Design review of the part shown in the three views and the two pictorial views. Dimensions are in mm from the part's minimum x, y and z. A direction names the side the tool comes from. Give positions to 0.01 mm unless a question says otherwise; leave off trailing zeros. Write each loop counter-clockwise with the first axis right and the second up, starting at its lowest first coordinate (ties: lowest second). Pieces come first, ordered by that corner, then holes. Notation, with made-up numbers: (27.5, 32) -> (59.5, 32) arc R27 ccw to (59.5, 64) -> close; hole circle Ø3 at (13, 13.25). An arc over 180 degrees is marked (long way). Use CSV: the item, a comma, the result in double quotes.
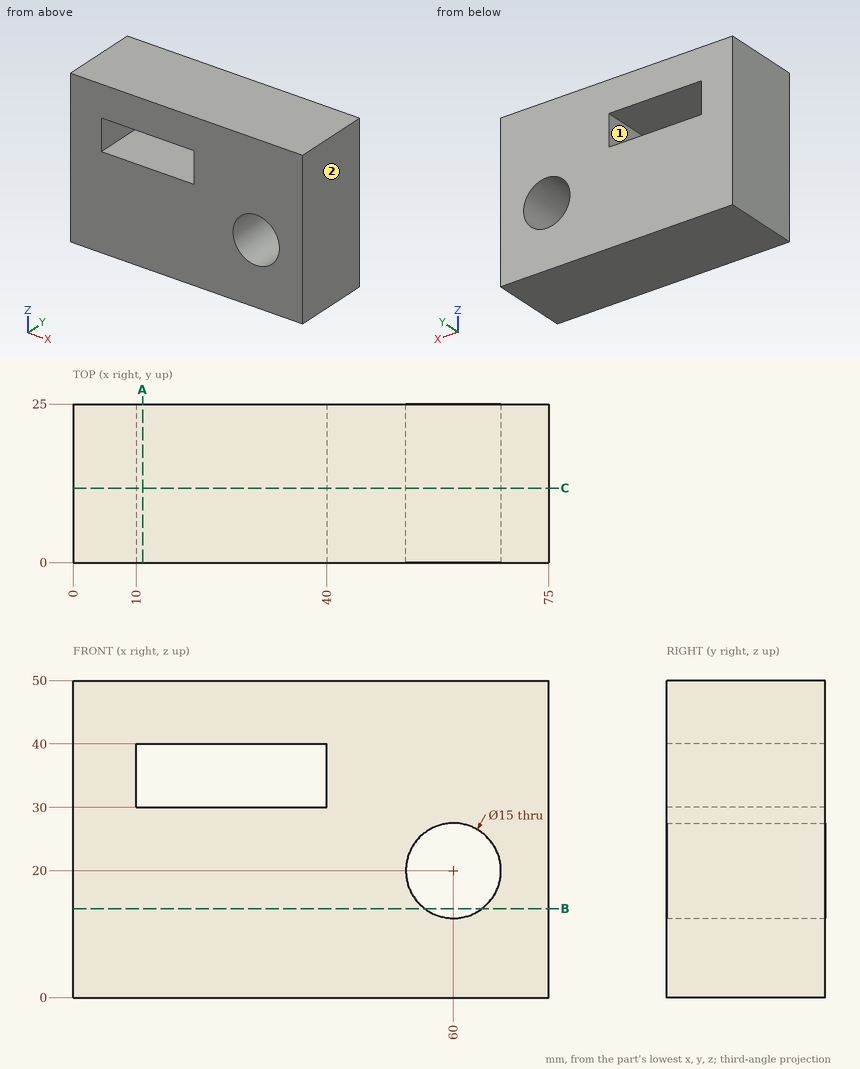
Q1. Insertion check: pin 1 (4 mm diameter, centred on x = 19.5, z = 7.5, fed in from -Y). The pin has a flat end and moves straight along its axis. Give the tip position at first contact, or say it passes through.
Derived:
pin 1,"stops at y = 0"
Q2. Consider section C-C (y = 11.75). Write out the cut boundary in (x, z).
Derived:
outline,"(0, 0) -> (75, 0) -> (75, 50) -> (0, 50) -> close; hole (10, 30) -> (40, 30) -> (40, 40) -> (10, 40) -> close; hole circle Ø15 at (60, 20)"
Q3. Machinability: for the marked faces 1 and 2, which of the approach directions +Z, -Z, +X, -X, +Y, -Y give a long, thin tool a straight path to every point of the face, cutting with its end or side? Answer none if there is none.
Derived:
face 1,"+Y, -Y"
face 2,"+Z, -Z, +X, +Y, -Y"
Q4. To check wall thickness, follow probe 1 along Z at (x, y) = (21, 21.25); probe 2 along Z at (x, y) = (60, 5.5); probe 3 along X at (y, z) = (19.5, 39). State the ranges of each line that lie inside material, in increasing order.
Derived:
probe 1,"z = 0 to 30, 40 to 50"
probe 2,"z = 0 to 12.5, 27.5 to 50"
probe 3,"x = 0 to 10, 40 to 75"
Q5. Consider section B-B (z = 14). Write out the cut boundary in (x, y).
Derived:
outline,"(0, 0) -> (55.5, 0) -> (55.5, 25) -> (0, 25) -> close; (64.5, 0) -> (75, 0) -> (75, 25) -> (64.5, 25) -> close"
Q6. Consider section A-A (x = 11). Write out the cut boundary in (y, z), then the cut area to 3 significant figures.
Derived:
outline,"(0, 0) -> (25, 0) -> (25, 30) -> (0, 30) -> close; (0, 40) -> (25, 40) -> (25, 50) -> (0, 50) -> close"
area,"1,000 mm2"
